Model file for the job. Use its own axes, mm. Coordinates: 2 decimals unless noted, no trailing zeros. Write each loop counter-clockwise with the first axis right and the second up, starting at its lowest first coordinate (ties: lowest second). Pieces come first, ordered by that corner, then holes.
Q1. Band-saw the part on C-C, the plane y = -5.25. State how many separate pieces and enclosed holes the cut face has, plus the area to 3 significant figures.
Q2. Band-saw the part on A-A, the plane x = 0. Write the cut outline in (y, z), plus the area to 3 significant figures.
Q3. Drill centre lines: probe 1 along Z at (x, y) = (0, -8.5); probe 2 along Z at (x, y) = (29.5, -4); probe 3 along X at (y, z) = (-13.5, 69). Where is each one in solid material? Low to high.
Q4. Pin check, flat tips, straight feed: P1, Ø5, axis at x = -75, y = -7.5, coming from the -Z side; P2, Ø6, axis at x = -58, y = -9, coming from the +Z side; P3, Ø1.5, axis at y = -6.5, z = -57.5, coming from the -X side. Stop position of each tip, or through.
Q5. Band-saw the part on D-D, the plane z = 63. Write the cut outline in (x, y), plus the area to 3 significant figures.
Q6. Band-saw the part on B-B, the plane z = 0. Write the cut outline in (x, y).
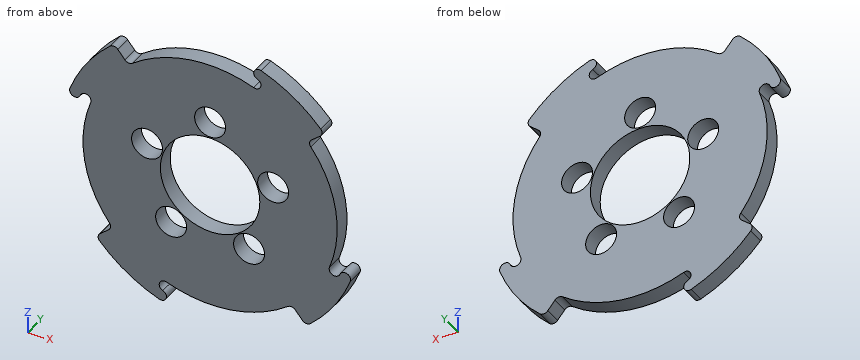
from build123d import *

# Parameters (mm, degrees)
F0_R     = 14
F0_R_2   = 45
F1_DEPTH = 15
F3_COUNT = 4
F4_R     = 14
F5_DEPTH = 15.001


# Not quite as in the source:
# - a feature names something its author has since deleted; it is built from what else it names


with BuildPart() as f1:
    # F0 (on Front) → F1 (new body)
    with BuildSketch(Plane.XZ):
        with BuildLine():
            ThreePointArc((-117.4615775982, 42.7525179157), (-111.0530137777, 45.740880303), (-108.0646513904, 39.3323164825))
            ThreePointArc((-108.0646513904, 39.3323164825), (-113.6444232454, -17.6052567496), (-91.0986302517, -70.1857504502))
            ThreePointArc((-91.0986302517, -70.1857504502), (-90.0886289945, -73.7767817278), (-91.8455022142, -77.0675270332))
            Line((-91.8455022142, -77.0675270332), (-99.5120922253, -83.500559884))
            ThreePointArc((-99.5120922253, -83.500559884), (-101.2865881138, -86.990889679), (-100.0019293376, -90.6896583342))
            ThreePointArc((-100.0019293376, -90.6896583342), (-75.2914558589, -112.0544362114), (-46.172719349, -126.8585038061))
            ThreePointArc((-46.172719349, -126.8585038061), (-39.7641555284, -123.8701414188), (-42.7525179157, -117.4615775982))
            ThreePointArc((-42.7525179157, -117.4615775982), (-45.740880303, -111.0530137777), (-39.3323164825, -108.0646513904))
            ThreePointArc((-39.3323164825, -108.0646513904), (17.6052567496, -113.6444232454), (70.1857504502, -91.0986302517))
            ThreePointArc((70.1857504502, -91.0986302517), (73.7767817278, -90.0886289945), (77.0675270332, -91.8455022142))
            Line((77.0675270332, -91.8455022142), (83.500559884, -99.5120922253))
            ThreePointArc((83.500559884, -99.5120922253), (86.990889679, -101.2865881138), (90.6896583342, -100.0019293376))
            ThreePointArc((90.6896583342, -100.0019293376), (112.0544362114, -75.2914558589), (126.8585038061, -46.172719349))
            ThreePointArc((126.8585038061, -46.172719349), (123.8701414188, -39.7641555284), (117.4615775982, -42.7525179157))
            ThreePointArc((117.4615775982, -42.7525179157), (111.0530137777, -45.740880303), (108.0646513904, -39.3323164825))
            ThreePointArc((108.0646513904, -39.3323164825), (113.6444232454, 17.6052567496), (91.0986302517, 70.1857504502))
            ThreePointArc((91.0986302517, 70.1857504502), (90.0886289945, 73.7767817278), (91.8455022142, 77.0675270332))
            Line((91.8455022142, 77.0675270332), (99.5120922253, 83.500559884))
            ThreePointArc((99.5120922253, 83.500559884), (101.2865881138, 86.990889679), (100.0019293376, 90.6896583342))
            ThreePointArc((100.0019293376, 90.6896583342), (75.2914558589, 112.0544362114), (46.172719349, 126.8585038061))
            ThreePointArc((46.172719349, 126.8585038061), (39.7641555284, 123.8701414188), (42.7525179157, 117.4615775982))
            ThreePointArc((42.7525179157, 117.4615775982), (45.740880303, 111.0530137777), (39.3323164825, 108.0646513904))
            ThreePointArc((39.3323164825, 108.0646513904), (-17.6052567496, 113.6444232454), (-70.1857504502, 91.0986302517))
            ThreePointArc((-70.1857504502, 91.0986302517), (-73.7767817278, 90.0886289945), (-77.0675270332, 91.8455022142))
            Line((-77.0675270332, 91.8455022142), (-83.500559884, 99.5120922253))
            ThreePointArc((-83.500559884, 99.5120922253), (-86.990889679, 101.2865881138), (-90.6896583342, 100.0019293376))
            ThreePointArc((-90.6896583342, 100.0019293376), (-112.0544362114, 75.2914558589), (-126.8585038061, 46.172719349))
            ThreePointArc((-126.8585038061, 46.172719349), (-123.8701414188, 39.7641555284), (-117.4615775982, 42.7525179157))
        make_face()
        with Locations((-35.2671151375, -48.5410196625)):
            Circle(F0_R, mode=Mode.SUBTRACT)
        with Locations((35.2671151375, -48.5410196625)):
            Circle(F0_R, mode=Mode.SUBTRACT)
        with Locations((-57.0633909777, 18.5410196625)):
            Circle(F0_R, mode=Mode.SUBTRACT)
        Circle(F0_R_2, mode=Mode.SUBTRACT)
        with Locations((57.0633909777, 18.5410196625)):
            Circle(F0_R, mode=Mode.SUBTRACT)
        with Locations((0, 60)):
            Circle(F0_R, mode=Mode.SUBTRACT)
    extrude(amount=F1_DEPTH)

    # F3: F1 ×4 about axis
    f3_axis = Axis((0, -15, 0), (0, -1, 0))


with BuildPart() as f1_1:
    add(f1.part)
    for i in range(1, F3_COUNT):
        add(f1.part.rotate(f3_axis, i * 360 / F3_COUNT))

    # F4 (on face) → F5 (cut, through all)
    with BuildSketch(Plane.XZ.offset(15)):
        with Locations((0, 60)):
            Circle(F4_R)
        with Locations((-57.0633909777, 18.5410196625)):
            Circle(F4_R)
        with Locations((-35.2671151375, -48.5410196625)):
            Circle(F4_R)
        with Locations((35.2671151375, -48.5410196625)):
            Circle(F4_R)
        with Locations((57.0633909777, 18.5410196625)):
            Circle(F4_R)
    extrude(amount=-F5_DEPTH, mode=Mode.SUBTRACT)


solid = f1_1.part
Answer sheet:
1. separate pieces: 1
1. enclosed holes: 6
1. area: 37,300 mm2
2. outline: (-15, -115) - (0, -115) - (0, -45) - (-15, -45) - close; (-15, 45) - (0, 45) - (0, 46) - (-15, 46) - close; (-15, 74) - (0, 74) - (0, 115) - (-15, 115) - close
2. area: 1,680 mm2
3. probe 1: z = -115 to -45, 45 to 46, 74 to 115
3. probe 2: z = -111.15 to -61.3, -35.78 to -33.98, 33.98 to 111.15
3. probe 3: x = -116.03 to -10.72, 10.72 to 92
4. P1: stops at z = -113.88
4. P2: stops at z = 101
4. P3: stops at x = -100.02
5. outline: (-119.4, -15) - (-13.67, -15) - (-13.67, 0) - (-119.4, 0) - close; (13.67, -15) - (96.21, -15) - (96.21, 0) - (13.67, 0) - close
5. area: 2,820 mm2
6. outline: (-115, -15) - (-45, -15) - (-45, 0) - (-115, 0) - close; (45, -15) - (115, -15) - (115, 0) - (45, 0) - close
